Part model, mm, in its own coordinate system. Round coordinates to 2 decimals unless told otherwise and drop trailing zeros. Write each loop counter-clockwise with the first axis right and the second up, starting at its lowest first coordinate (ties: lowest second). Pieces come first, ordered by that corner, then holes.
```python
from build123d import *

# Parameters (mm, degrees)
BOSS_EXTRUDE1_DEPTH = 2


with BuildPart() as part:
    # Sketch1 → Boss-Extrude1 (new body)
    with BuildSketch(Plane.XY):
        with BuildLine():
            Line((-160.973915689, -6.861918673), (6.826084311, -6.861918673))
            Line((6.826084311, -6.861918673), (6.826084311, -11.861918673))
            ThreePointArc((6.826084311, -11.861918673), (3.897152123, -18.932986485), (-3.173915689, -21.861918673))
            Line((-3.173915689, -21.861918673), (-170.973915689, -21.861918673))
            Line((-170.973915689, -21.861918673), (-170.973915689, -16.861918673))
            ThreePointArc((-170.973915689, -16.861918673), (-168.0449835, -9.790850861), (-160.973915689, -6.861918673))
        make_face()
    extrude(amount=BOSS_EXTRUDE1_DEPTH)


solid = part.part
```
Q1. Cut at B-B on y = -10. Write the cut outline in (x, z).
Values follow:
outline: (-168.25, 0) - (6.83, 0) - (6.83, 2) - (-168.25, 2) - close
Q2. Wall check: L1, parallel to X at y = -18, z = 1.3; L2, parallel to X at y = -14.25, z = 1.4. Give the ranges that are in metal, low to high.
Values follow:
L1: x = -170.97 to 4.72
L2: x = -170.63 to 6.54
Q3. Cut at C-C on y = -19.25. Write the cut outline in (x, z), plus the area to 3 significant figures.
Values follow:
outline: (-170.97, 0) - (3.57, 0) - (3.57, 2) - (-170.97, 2) - close
area: 349 mm2
Q4. Cut at A-A on z = 0.65. Write the cut outline in (x, y).
Values follow:
outline: (-170.97, -21.86) - (-3.17, -21.86) arc R10 ccw to (6.83, -11.86) - (6.83, -6.86) - (-160.97, -6.86) arc R10 ccw to (-170.97, -16.86) - close
